Source: CAD feature listing. Evaluate the final solid. Frame: model axes, mm. Face numbers are marked on the shaded views. A direction names the side the tool comes from. Coordinates: 2 decimals unless noted, no trailing zeros. Order: outer loops, then holes, each group sorted by start corner. A loop starts at its lowest first (then second) coordinate and runs counter-clockwise, first axis right, second up.
```python
from build123d import *

# Parameters (mm, degrees)
SKETCH1_W                      = 11.1
SKETCH1_H                      = 12.7
SKETCH2_R                      = 4
BOSS_EXTRUDE1_DEPTH            = 2.525
SKETCH3_R                      = 4
BOSS_EXTRUDE2_DEPTH            = 2.525
M2_5_CLEARANCE_HOLE1_D         = 2.705
M2_5_CLEARANCE_HOLE1_DEPTH     = 15.225
F_4_9_4_9_DIAMETER_HOLE1_D     = 4.9
F_4_9_4_9_DIAMETER_HOLE1_DEPTH = 17.75


with BuildPart() as part:
    # Sketch1 → Revolve1 (revolve)
    with BuildSketch(Plane(origin=(0, 0, 0), x_dir=(1, 0, 0), z_dir=(0, 1, 0))):
        with Locations((5.55, 0)):
            Rectangle(SKETCH1_W, SKETCH1_H)
    revolve(axis=Axis((0, 0, -6.35), (0, 0, 1)))

    # Sketch2 → Boss-Extrude1 (add)
    with BuildSketch(Plane(origin=(0, 0, -6.35), x_dir=(-1, 0, 0), z_dir=(0, 0, -1))):
        Circle(SKETCH2_R)
    extrude(amount=BOSS_EXTRUDE1_DEPTH)

    # Sketch3 → Boss-Extrude2 (add)
    with BuildSketch(Plane.XY.offset(6.35)):
        Circle(SKETCH3_R)
    extrude(amount=BOSS_EXTRUDE2_DEPTH)

    # M2.5 Clearance Hole1
    with Locations(Plane.XY.offset(6.35)):
        with Locations((5.656854249, 5.656854249), (-5.656854249, 5.656854249), (-5.656854249, -5.656854249), (5.656854249, -5.656854249)):
            Hole(M2_5_CLEARANCE_HOLE1_D / 2, depth=M2_5_CLEARANCE_HOLE1_DEPTH)

    # Ø4.9 (4.9) Diameter Hole1
    with Locations(Plane(origin=(0, 0, -8.875), x_dir=(-1, 0, 0), z_dir=(0, 0, -1))):
        with Locations((0, 0)):
            Hole(F_4_9_4_9_DIAMETER_HOLE1_D / 2, depth=F_4_9_4_9_DIAMETER_HOLE1_DEPTH)


solid = part.part
```
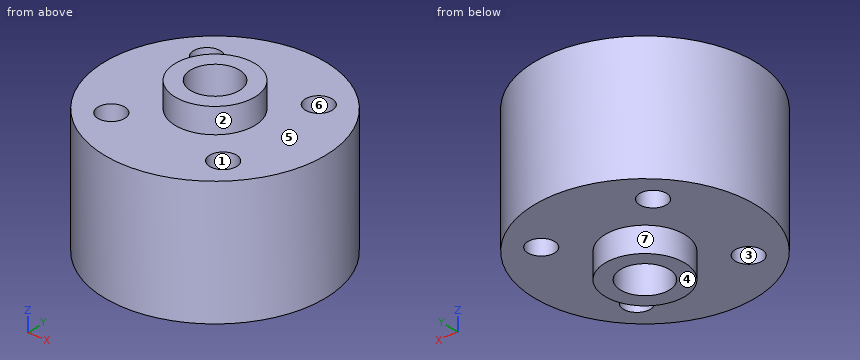
1. Contact query for flat-ended pins moving along their axis: P1, Ø5, axis at x = -5, z = 2, coming from the -Y side; P2, Ø4, axis at y = -7.5, z = -1, coming from the +X side; P3, Ø4, axis at x = 6.5, z = 1.5, coming from the +Y side. Output: stop coordinate, or through.
2. Material intervals for line 1 along Y through (x, z) = (6, -2.75); line 2 along Z through (x, y) = (-6.25, 0.5), sorted ascending.
3. Section query A-A, the plane x = 0. Output: boundary loops of the cut face in (y, z) (3 decimals), plus the area to 3 significant figures.
4. Draft query along Y for the marked faces 1, 2, 3 and 4. Return one class per face: +Y half, -Y half, draft (parallel to the pull), parting line (faces both ways), or undercut.
5. Section query C-C, the plane y = -5.25. Output: boundary loops of the cut face in (x, z).
6. Access query for the marked faces 5, 6 and 7. Directions: +Z, -Z, +X, -X, +Y, -Y. A direction counts if a zero-diameter tool reaches every point of the face in a straight line with its end or side. Return the directions, or none.
Answer key:
1. P1: stops at y = -10.81
1. P2: stops at x = 9.64
1. P3: stops at y = 10.15
2. line 1: y = -9.34 to -6.97, -4.35 to 4.35, 6.97 to 9.34
2. line 2: z = -6.35 to 6.35
3. outline: (-11.1, -6.35) - (-4, -6.35) - (-4, -8.875) - (-2.45, -8.875) - (-2.45, 8.875) - (-4, 8.875) - (-4, 6.35) - (-11.1, 6.35) - close; (2.45, -8.875) - (4, -8.875) - (4, -6.35) - (11.1, -6.35) - (11.1, 6.35) - (4, 6.35) - (4, 8.875) - (2.45, 8.875) - close
3. area: 235 mm2
4. face 1: undercut
4. face 2: parting line
4. face 3: undercut
4. face 4: draft
5. outline: (-9.78, -6.35) - (-6.95, -6.35) - (-6.95, 6.35) - (-9.78, 6.35) - close; (-4.37, -6.35) - (4.37, -6.35) - (4.37, 6.35) - (-4.37, 6.35) - close; (6.95, -6.35) - (9.78, -6.35) - (9.78, 6.35) - (6.95, 6.35) - close
6. face 5: +Z
6. face 6: +Z, -Z
6. face 7: -Z
